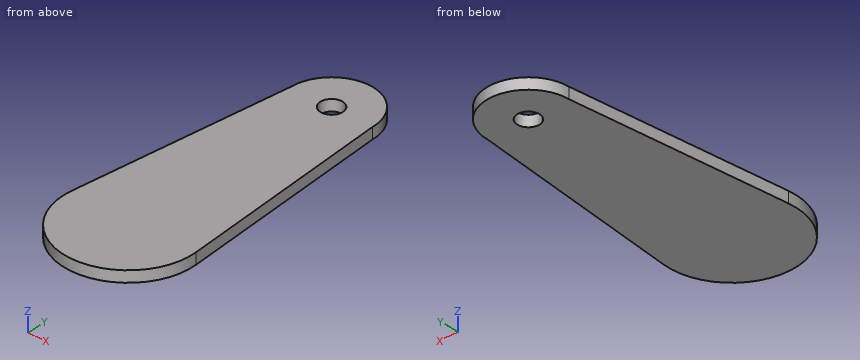
```python
from build123d import *

# Parameters (mm, degrees)
F0_R     = 2
F1_DEPTH = 2


with BuildPart() as f1:
    # F0 (on Top) → F1 (new body)
    with BuildSketch(Plane.XY):
        with BuildLine():
            Line((-7.5, 40.559527), (-11.442887, 1.144696))
            ThreePointArc((-11.442887, 1.144696), (0, -11.5), (11.442887, 1.144696))
            Line((11.442887, 1.144696), (7.5, 40.559527))
            ThreePointArc((7.5, 40.559527), (0, 48.059527), (-7.5, 40.559527))
        make_face()
        with Locations((0, 40.559527)):
            Circle(F0_R, mode=Mode.SUBTRACT)
    extrude(amount=F1_DEPTH)


solid = f1.part
```
Could you check a few things on this model? Use its own coordinates, in mm. Coordinates: 2 decimals unless noted, no trailing zeros. Loops run counter-clockwise (first coordinate to the right, second up) from the corner with the lowest first, then second, coordinate; pieces in that order, holes last. Notation, with made-up numbers: M 29.25,6 L 72.25,6 A24 ccw 72.25,27 Z; hole C 60,-22 d6. An arc over 180 degrees is marked long. Put each result on its own line as item: value. Start each with the question number.
(1) Suppose I cut it at A-A on x = 0. Please give me the cut outline in (y, z), then the cut area to 3 significant figures.
(2) Suppose I cut it at D-D on x = 8.5. Please give me the cut outline in (y, z).
(3) Suppose I cut it at C-C on y = 44. Please give me the cut outline in (x, z), then the cut area to 3 significant figures.
(4) Suppose I cut it at B-B on z = 1.5. Please give me the cut outline in (x, y), then the cut area to 3 significant figures.
(5) I need wall thicknesses on line 1 (Y direction, x = 0, z = 0.75); line 2 (X direction, y = 40.5, z = 1.05); line 3 (X direction, y = 42, z = 0.6). Which ranges of each line are inside material? Lowest first, please. Write a range as from..to.
Solutions:
1. outline: M -11.5,0 L 38.56,0 L 38.56,2 L -11.5,2 Z; M 42.56,0 L 48.06,0 L 48.06,2 L 42.56,2 Z
1. area: 111 mm2
2. outline: M -7.75,0 L 30.56,0 L 30.56,2 L -7.75,2 Z
3. outline: M -6.66,0 L 6.66,0 L 6.66,2 L -6.66,2 Z
3. area: 26.7 mm2
4. outline: M -11.44,1.14 A11.5 ccw long 11.44,1.14 L 7.5,40.56 A7.5 ccw -7.5,40.56 Z; hole C 0,40.56 d4
4. area: 1,060 mm2
5. line 1: y = -11.5..38.56, 42.56..48.06
5. line 2: x = -7.51..-2, 2..7.51
5. line 3: x = -7.36..-1.39, 1.39..7.36
